For this review, take the finished solid that the model builds, in its own axes (mm). A direction names the side the tool comes from. Coordinates: 2 decimals unless noted, no trailing zeros. Write each loop counter-clockwise with the first axis right and the second up, starting at its lowest first coordinate (ties: lowest second). Pieces come first, ordered by that corner, then holes.
```python
from build123d import *

# Parameters (mm, degrees)
SKETCH1_R                       = 5
SKETCH1_R_2                     = 4
BOSS_EXTRUDE1_DEPTH             = 150
CUT_EXTRUDE1_DEPTH              = 21
CUT_EXTRUDE1_DEPTH_BACK         = 21
SKETCH2_R                       = 1.5
BOSS_EXTRUDE2_START             = 10
SKETCH3_R                       = 5
BOSS_EXTRUDE2_DEPTH             = 60
BOSS_EXTRUDE2_DIRECTION_2_REACH = 162.167
SKETCH4_R                       = 3
CUT_EXTRUDE2_DEPTH              = 20


with BuildPart() as part:
    # Sketch1 → Boss-Extrude1 (new body)
    with BuildSketch(Plane.XY):
        Circle(SKETCH1_R)
        Circle(SKETCH1_R_2, mode=Mode.SUBTRACT)
    extrude(amount=BOSS_EXTRUDE1_DEPTH)

    # Sketch2 → Cut-Extrude1 (cut, two sides: drawn at the far end of the back side and taken through both)
    with BuildSketch(Plane(origin=(0, 0, 0), x_dir=(1, 0, 0), z_dir=(0, 1, 0)).offset(-CUT_EXTRUDE1_DEPTH_BACK)):
        with Locations(Location((0, -142, 0), (0, 0, 90))):
            Circle(SKETCH2_R)
        with Locations(Location((0, -8, 0), (0, 0, 90))):
            Circle(SKETCH2_R)
    extrude(amount=CUT_EXTRUDE1_DEPTH + CUT_EXTRUDE1_DEPTH_BACK, mode=Mode.SUBTRACT)

    # Sketch3 → Boss-Extrude2 (add)
    with BuildSketch(Plane(origin=(0, 0, 0), x_dir=(1, 0, 0), z_dir=(0, 1, 0)).offset(BOSS_EXTRUDE2_START)):
        with Locations(Location((0, -105, 0), (0, 0, 270))):
            Circle(SKETCH3_R)
    extrude(amount=BOSS_EXTRUDE2_DEPTH)

    # Sketch3 → Boss-Extrude2 direction 2 (add, up to next)
    with BuildSketch(Plane(origin=(0, 0, 0), x_dir=(1, 0, 0), z_dir=(0, 1, 0)).offset(BOSS_EXTRUDE2_START), mode=Mode.PRIVATE) as boss_extrude2_direction_2_sk1:
        with Locations(Location((0, -105, 0), (0, 0, 270))):
            Circle(SKETCH3_R)
    boss_extrude2_direction_2_tool1 = extrude(boss_extrude2_direction_2_sk1.sketch, amount=-BOSS_EXTRUDE2_DIRECTION_2_REACH, mode=Mode.PRIVATE) - part.part
    add(boss_extrude2_direction_2_tool1.solids().sort_by_distance((0, 10, 105))[0])

    # Sketch4 → Cut-Extrude2 (cut)
    with BuildSketch(Plane(origin=(0, 70, 0), x_dir=(1, 0, 0), z_dir=(0, 1, 0))):
        with Locations(Location((0, -105, 0), (0, 0, 270))):
            Circle(SKETCH4_R)
    extrude(amount=-CUT_EXTRUDE2_DEPTH, mode=Mode.SUBTRACT)


solid = part.part
```
Q1. For probe 1 along X at (y, z) = (4, 142); probe 2 along Y at (x, z) = (0.5, 39), list the stretches that pass through material, from the lowest coordinate up.
Ans:
probe 1: x = -3 to -1.5, 1.5 to 3
probe 2: y = -4.97 to -3.97, 3.97 to 4.97
Q2. Tool access review of faces 5 (the cylindrical face through (-1.8, 60.1, 102.6)), 6 (the cylindrical face through (1.846, -3.549, 73.95)): name each direction out of +Z, -Z, +X, -X, +Y, -Y from which nothing blocks a thin tool from reaching the whole face with its end or side.
Ans:
face 5: +Y
face 6: +Z, -Z
Q3. Add section A-A (x = 0). Give the number of separate pieces and of enclosed holes in the cut face, then the cut area to 3 significant figures.
Ans:
separate pieces: 6
enclosed holes: 0
area: 818 mm2
Q4. Clearance check with flat-ended pins moving along their axes: pin 1 Ø1.5 at (x, z) = (-2, 32) entering from +Y; pin 2 Ø5 at (x, z) = (0, 142) entering from -Y; pin 3 Ø5 at (x, z) = (0, 8) entering from +Y; pin 4 Ø3 at (y, z) = (34, 100) entering from -X. State where each tip first meets the part, or that it passes through.
Ans:
pin 1: stops at y = 4.84
pin 2: stops at y = -5
pin 3: stops at y = 5
pin 4: stops at x = -3.57
Q5. Add section B-B (z = 105). State the section outline as (x, y) points.
Ans:
outline: (-5, 0) arc R5 ccw to (5, 0) - (5, 70) - (3, 70) - (3, 50) - (-3, 50) - (-3, 70) - (-5, 70) - close; hole circle Ø8 at (0, 0)
Q6. Draft analysis for pull direction X (two halves, no side actions). For faces 1 (the cylindrical face through (2.307, -4.436, 73.95)), 2 (the cylindrical face through (1.33, -4.37, 7.31)), 3 (the flat face through (-3.3, 70, 104.9)), 4 (the cylindrical face through (1.33, -4.37, 141.31)), state which applies: +X half, -X half, draft (parallel to the pull), parting line (faces both ways), or undercut.
Ans:
face 1: parting line
face 2: undercut
face 3: draft
face 4: undercut
Q7. Add section D-D (z = 142). State the section outline as (x, y) points, then the cut area to 3 significant figures.
Ans:
outline: (-1.5, -4.77) - (-1.5, -3.71) arc R4 cw to (-1.5, 3.71) - (-1.5, 4.77) arc R5 ccw to start; (1.5, -4.77) arc R5 ccw to (1.5, 4.77) - (1.5, 3.71) arc R4 cw to (1.5, -3.71) - close
area: 22.2 mm2
Q8. Add section C-C (y = 58.5). State the section outline as (x, z) points.
Ans:
outline: circle Ø10 at (0, 105); hole circle Ø6 at (0, 105)
